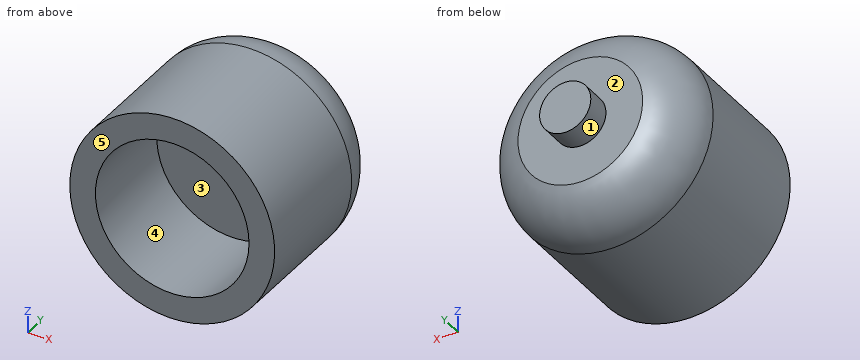
```python
from build123d import *

# Parameters (mm, degrees)
SKETCH3_R          = 300
CUT_EXTRUDE1_DEPTH = 400


with BuildPart() as part:
    # Sketch1 → Revolve2 (revolve)
    with BuildSketch(Plane.XY):
        with BuildLine():
            Line((0, 266.536964981), (0, -433.463035019))
            Line((0, -433.463035019), (-400, -433.463035019))
            Line((-400, -433.463035019), (-400, 68.62497771))
            ThreePointArc((-400, 68.62497771), (-356.145251984, 194.783226442), (-243.492938859, 266.536964981))
            Line((-243.492938859, 266.536964981), (-100, 266.536964981))
            Line((-100, 266.536964981), (-100, 364.980544747))
            Line((-100, 364.980544747), (0, 364.980544747))
            Line((0, 364.980544747), (0, 266.536964981))
        make_face()
    revolve(axis=Axis((0, 266.536964981, 0), (0, -1, 0)))

    # Sketch3 → Cut-Extrude1 (cut)
    with BuildSketch(Plane.XZ.offset(433.463035019)):
        Circle(SKETCH3_R)
    extrude(amount=-CUT_EXTRUDE1_DEPTH, mode=Mode.SUBTRACT)


solid = part.part
```
Input: part model. Units: mm. Frame: model coordinates. Face numbers are marked on the shaded views. A direction names the side the tool comes from. Give positions to 0.01 mm unless a question says otherwise; leave off trailing zeros. Order: outer loops, then holes, each group sorted by start corner. A loop starts at its lowest first (then second) coordinate and runs counter-clockwise, first axis right, second up.
1. Cut plane B-B (y = 317.5). Return loops of the section in (x, z), and give its area (3 significant figures).
Computed:
outline: circle Ø200 at (0, 0)
area: 31,400 mm2
2. Set-up query: the marked faces 4 and 5. Return all of +Z, -Z, +X, -X, +Y, -Y with unobstructed straight access to the full face (end or side cutting, diameter ignored); none if empty.
Computed:
face 4: -Y
face 5: +Z, -Z, +X, -X, -Y
3. Draft query along X for the marked faces 1, 2 and 3. Return one class per face: released by +X, released by -X, zero draft, split by the parting line, or undercut.
Computed:
face 1: split by the parting line
face 2: zero draft
face 3: undercut
4. Pin query (flat end, axial travel): pin 1 Ø6 at (y, z) = (-138.5, 101.5) entering from -X; pin 2 Ø2 at (x, y) = (294.5, -216.5) entering from +Z; pin 3 Ø10 at (x, y) = (-119, -99.5) entering from -Z. Return the tip coordinate at first contact, or that it passes through.
Computed:
pin 1: stops at x = -387.68
pin 2: stops at z = 271.77
pin 3: stops at z = -383.41
5. Line query: probe 1 along Z at (x, y) = (0, -282.5); probe 2 along Z at (x, y) = (3.5, 289.5); probe 3 along Y at (x, z) = (231, 56). Output: solid intervals per line, ascending.
Computed:
probe 1: z = -400 to -300, 300 to 400
probe 2: z = -99.94 to 99.94
probe 3: y = -33.46 to 266.54
6. Cut plane A-A (y = -370). Return loops of the section in (x, z).
Computed:
outline: circle Ø800 at (0, 0); hole circle Ø600 at (0, 0)
